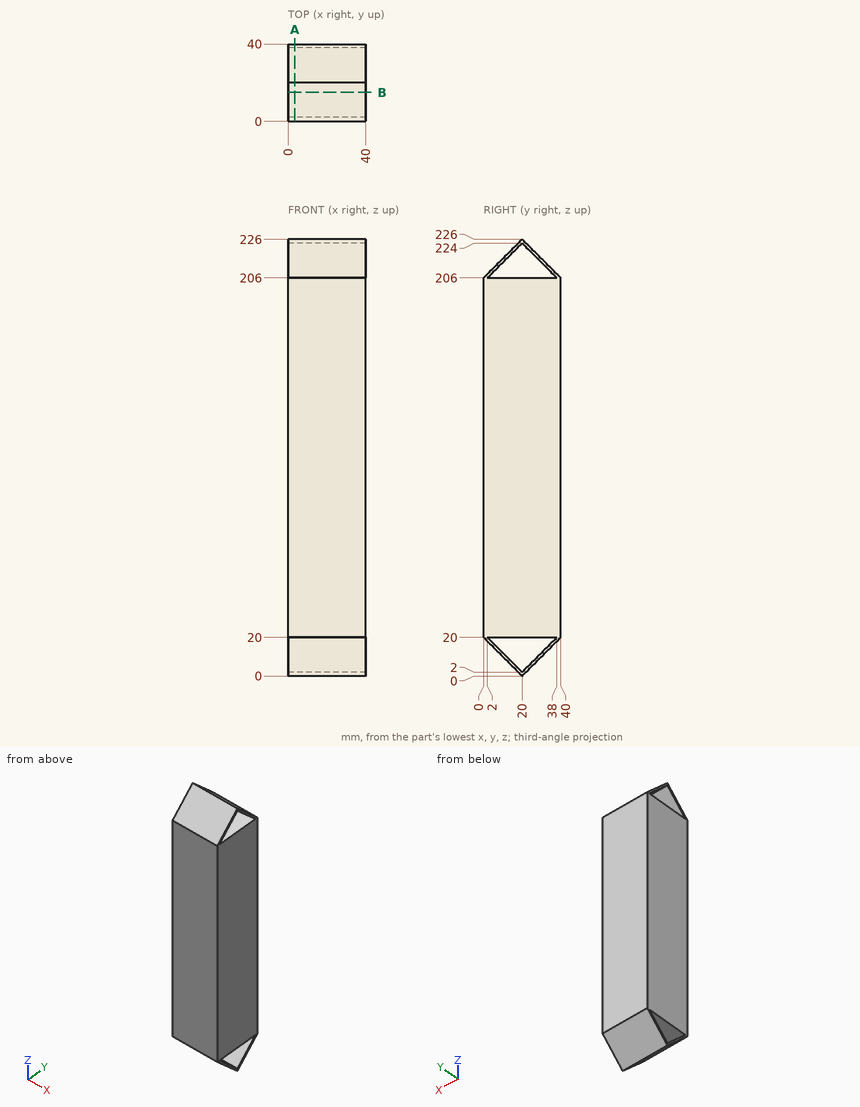
Geometry check sheet. Reference: drawing and pictorial views, mm from the part's lowest x, y, z. Give positions to 0.01 mm unless a question says otherwise; leave off trailing zeros. Order: outer loops, then holes, each group sorted by start corner. A loop starts at its lowest first (then second) coordinate and runs counter-clockwise, first axis right, second up. Notation, with made-up numbers: M 7,78 L 52,78 A37 cw 52,114 Z; hole C 57.5,-38.75 d4. An arc over 180 degrees is marked long. Answer in a Markdown table with one row per item. Add a question column.
Item 1: Scan lines: probe 1 along Z at (x, y) = (13.5, 17); probe 2 along Z at (x, y) = (38.5, 25); probe 3 along Y at (x, z) = (28.5, 212.5). Record each from-to range of solid material in increasing order. Write a range as from..to.
Item 2: Gauge pin test, flat ends, axial feed: pin 1 (1.5 mm diameter, centred on x = 9.5, y = 12.5, fed in from -Z); pin 2 (8 mm diameter, centred on x = 13, y = 29, fed in from -Z). Record the tip position at first contact, or that the pin passes through.
Item 3: Section check A-A, the plane x = 3.5. Enter the section's corners in (y, z).
Item 4: Section check B-B, the plane y = 15. Enter the section's corners in (x, z).
Filled sheet:
| question | item | result |
|---|---|---|
| 1 | probe 1 | z = 3..5, 20..206, 221..223 |
| 1 | probe 2 | z = 5..7, 20..206, 219..221 |
| 1 | probe 3 | y = 6.5..8.5, 31.5..33.5 |
| 2 | pin 1 | stops at z = 6.75 |
| 2 | pin 2 | stops at z = 5 |
| 3 | outline | M 0,20 L 20,0 L 40,20 L 40,206 L 20,226 L 0,206 Z; hole M 2,20 L 20,2 L 38,20 Z; hole M 2,206 L 38,206 L 20,224 Z |
| 4 | outline | M 0,5 L 40,5 L 40,7 L 0,7 Z; M 0,20 L 40,20 L 40,206 L 0,206 Z; M 0,219 L 40,219 L 40,221 L 0,221 Z |
